Verification items for the finished model (mm, model axes). A direction names the side the tool comes from. Give positions to 0.01 mm unless a question says otherwise; leave off trailing zeros. Order: outer loops, then holes, each group sorted by start corner. A loop starts at its lowest first (then second) coordinate and runs counter-clockwise, first axis right, second up. Notation, with made-up numbers: (89.5, 56.25) - (114.5, 56.25) arc R18 ccw to (114.5, 64.25) - close; hole circle Ø4 at (-11.75, 84.25). An arc over 180 degrees is marked (long way). Answer as a JSON object with one key per item and string values. Group by question number.
(1) Section check D-D (x = 79). Record the boundary of the cut face in (y, z).
(2) Thickness scan on line 1 (Z direction, x = 384, y = 75); line 2 (Y direction, x = 166.5, z = -29.5); line 3 (Y direction, x = 413.5, z = -49). Record the ranges inside material, lowest first.
(3) Section check C-C (y = 30.5). Record the boundary of the cut face in (x, z), then the cut area to 3 significant figures.
(4) Mould release check, pull along Z, two halves, no side actions. Record for faces 4 (the face through (0, 155, 0)), 5 (the face through (247, 69, 60)), 6 (the face through (303, 66, -45)): +Z half, -Z half, draft (parallel to the pull), parting line (faces both ways), or undercut.
(5) Access from +Z, -Z, +X, -X, +Y, -Y to the whole of each face (thin tool, end or side, straight path). Record for faces 1 (the face through (11.923, 147.395, 3.755)), 2 (the face through (11.923, -7.395, -3.755)), 3 (the face through (303, 64, 45)).
(6) Section check B-B (z = 0). Record the boundary of the cut face in (x, y).
(7) Depth check by flat-ended pin: pin 1 Ø4 at (x, z) = (273, -31) entering from +Y; pin 2 Ø2 at (x, z) = (217, -36.5) entering from -Y. Enter the tip coordinate at first touch or a pass-through.
(8) Section check A-A (x = 146). Record the boundary of the cut face in (y, z).
Autodesk Inventor part; units mm, degrees
ref_plane "YZ Plane" through (0, 0, 0) normal (1, 0, 0) x (0, 1, 0)
ref_plane "XZ Plane" through (0, 0, 0) normal (0, 1, 0) x (-1, 0, 0)
ref_plane "XY Plane" through (0, 0, 0) normal (0, 0, 1) x (1, 0, 0)
sketch "Szkic1" plane through (0, 0, 0) normal (0, 1, 0) x (-1, 0, 0)
  circle A0 centre (0, 0) radius 60
  line L0 (0, 60) -> (-500, 60)
  line L1 (-500, 60) -> (-500, -60)
  line L2 (-500, -60) -> (0, -60)
  line L3 (0, -60) -> (0, 60)
  point P0 (0, -60)
  dimension "d0" = 120
  dimension "d1" = 500
  dimension "d2" = 120
extrude "Wyciągnięcie proste1" add sketch "Szkic1" along normal blind 140
sketch "Szkic2" plane through (0, 140, 0) normal (0, 1, 0) x (1, 0, 0)
  circle A0 centre (0, 0) radius 12.5
  dimension "d5" = 25
extrude "Wyciągnięcie proste2" add sketch "Szkic2" along normal blind 15
sketch "Szkic3" plane through (0, 0, 0) normal (0, -1, 0) x (1, 0, 0)
  circle A0 centre (0, 0) radius 12.5
  dimension "d8" = 25
extrude "Wyciągnięcie proste3" add sketch "Szkic3" along normal blind 15
sketch "Szkic4" plane through (500, 0, 60) normal (1, 0, 0) x (0, 0, -1)
  line L0 (0, 0) -> (0, 140)
  line L1 (0, 140) -> (120, 140)
  line L2 (120, 0) -> (120, 140)
  line L3 (0, 0) -> (120, 0)
  line L4 (15, 125) -> (105, 125)
  line L5 (105, 125) -> (105, 5)
  line L6 (105, 5) -> (15, 5)
  line L7 (15, 5) -> (15, 125)
  line L8 (15, 125) -> (105, 5) construction
  line L9 (105, 125) -> (15, 5) construction
  point P0 (60, 0)
  point P1 (60, 65)
  dimension "d11" = 90
  dimension "d12" = 120
  dimension "d13" = 15
  dimension "d14" = 15
extrude "Wyciągnięcie proste4" cut sketch "Szkic4" against normal blind 400 contours L4 L5 L6 L7
equation "\"PromieńGięcia\" = Grubość"
equation "\"SzerokośćGięciaPodcięcia\" = Grubość"
equation "\"GłębokośćGięciaPodcięcia\" = 0.5 * Grubość"
equation "\"RozmiarPodcięciaNarożnika\" = 4 * Grubość"
equation "\"MinimalnaPozostałość\" = 2 * Grubość"
equation "\"PromieńPrzejścia\" = PromieńGięcia"
equation "\"Rozmiar_promienia_Jacobiego\" = PromieńGięcia"
equation "\"Wielk_odstępu\" = Grubość"
properties part number "czesc2"
Solutions:
{
 "1": {"outline": "(0, -60) - (140, -60) - (140, 60) - (0, 60) - close"},
 "2": {"line 1": "z = -60 to -45, 45 to 60", "line 2": "y = 0 to 5, 125 to 140", "line 3": "y = 0 to 140"},
 "3": {"outline": "(0, -60) - (500, -60) - (500, -45) - (100, -45) - (100, 45) - (500, 45) - (500, 60) - (0, 60) arc R60 ccw to start", "area": "29,700 mm2"},
 "4": {"face 4": "draft", "face 5": "+Z half", "face 6": "undercut"},
 "5": {"face 1": "+Y", "face 2": "-Y", "face 3": "+X"},
 "6": {"outline": "(-60, 0) - (-12.5, 0) - (-12.5, -15) - (12.5, -15) - (12.5, 0) - (500, 0) - (500, 5) - (100, 5) - (100, 125) - (500, 125) - (500, 140) - (12.5, 140) - (12.5, 155) - (-12.5, 155) - (-12.5, 140) - (-60, 140) - close"},
 "7": {"pin 1": "stops at y = 140", "pin 2": "stops at y = 0"},
 "8": {"outline": "(0, -60) - (140, -60) - (140, 60) - (0, 60) - close; hole (5, -45) - (125, -45) - (125, 45) - (5, 45) - close"}
}
